Geometry: final body of the model. Coordinates: model frame, mm. A direction names the side the tool comes from. Round coordinates to 2 decimals unless told otherwise and drop trailing zeros. Loops run counter-clockwise (first coordinate to the right, second up) from the corner with the lowest first, then second, coordinate; pieces in that order, holes last. Notation, with made-up numbers: (24, 79.5) - (50, 79.5) arc R20 cw to (50, 87.5) - close; hole circle Ø7 at (3, 66). An arc over 180 degrees is marked (long way). Return JSON: item names as keys, results as strings. Group by question number.
1. Draft query along X for faces 1 (the face through (-11.99, 0.53, 11.75)), 2 (the face through (-2, 14, 13)), 3 (the face through (138.75, 4, 12)). Return one class per face: +X half, -X half, draft (parallel to the pull), parting line (faces both ways), or undercut.
2. Section B-B on x = -62.5. Return loops of the section in (y, z).
3. Section A-A on z = 10.1. Return loops of the section in (x, y), and give its area (3 significant figures).
4. First-contact query: pin 1 Ø2 at (x, z) = (31.5, 9.5) entering from -Y; pin 2 Ø2 at (x, y) = (-41.25, -58) entering from -Z; pin 3 Ø1.3 at (x, z) = (52, 8.5) entering from +Y. Flat tips, straight axial feed; report the tip coordinate or a pass-through.
5. Material intervals for probe 1 along X at (y, z) = (58, 11.75); probe 2 along Y at (x, z) = (-41.25, 11.7); probe 3 along Y at (x, z) = (-21, 7.35), sorted ascending.
6. Section C-C on y = 23. Return loops of the section in (x, z), and give its area (3 significant figures).
7. Set-up query: faces 4 (the face through (-2, 51, 11.5)), 5 (the face through (-138.75, 4, 12)), 6 (the face through (-2, 18, 11.5)), 7 (the face through (-2, -50, 11.5)). Return all of +Z, -Z, +X, -X, +Y, -Y with unobstructed straight access to the full face (end or side cutting, diameter ignored); none if empty.
from build123d import *

# Parameters (mm, degrees)
SKETCH017_W     = 277.5
SKETCH017_H     = 121
PAD007_DEPTH    = 1.5
SKETCH018_R     = 0.9
POCKET006_DEPTH = 1.501
SKETCH025_W     = 277.5
SKETCH025_H     = 2
PAD009_DEPTH    = 4.5
SKETCH026_R     = 12
POCKET007_DEPTH = 6.001
CHAMFER_SIZE    = 1


with BuildPart() as part:
    # Sketch017 → Pad007 (new body)
    with BuildSketch(Plane.XY.offset(13)):
        Rectangle(SKETCH017_W, SKETCH017_H)
    extrude(amount=-PAD007_DEPTH)

    # Sketch018 (on Face6 of Pad007) → Pocket006 (cut, through all)
    with BuildSketch(Plane(origin=(0, 0, 11.5), x_dir=(1, 0, 0), z_dir=(0, 0, -1))):
        with Locations((-135.25, 58)):
            Circle(SKETCH018_R)
        with Locations((-41.25, 58)):
            Circle(SKETCH018_R)
        with Locations((-31.25, 58)):
            Circle(SKETCH018_R)
        with Locations((43.75, 58)):
            Circle(SKETCH018_R)
        with Locations((135.25, 58)):
            Circle(SKETCH018_R)
        with Locations((135.25, -58)):
            Circle(SKETCH018_R)
        with Locations((43.75, -58)):
            Circle(SKETCH018_R)
        with Locations((-31.25, -58)):
            Circle(SKETCH018_R)
        with Locations((-41.25, -58)):
            Circle(SKETCH018_R)
        with Locations((-135.25, -58)):
            Circle(SKETCH018_R)
    extrude(amount=-POCKET006_DEPTH, mode=Mode.SUBTRACT)

    # Sketch025 (on Face5 of Pocket006) → Pad009 (join)
    with BuildSketch(Plane(origin=(0, 0, 11.5), x_dir=(1, 0, 0), z_dir=(0, 0, -1))):
        with Locations((0, 39.5)):
            Rectangle(SKETCH025_W, SKETCH025_H)
        with Locations((0, -39.5)):
            Rectangle(SKETCH025_W, SKETCH025_H)
    extrude(amount=PAD009_DEPTH)

    # Sketch026 (on Face2 of Pad009) → Pocket007 (cut, through all)
    with BuildSketch(Plane.XY.offset(13)):
        Circle(SKETCH026_R)
    extrude(amount=-POCKET007_DEPTH, mode=Mode.SUBTRACT)

    # Chamfer
    chamfer_edges = [part.edges().sort_by_distance(p)[0] for p in [
        (134.35, -58, 13),
        (42.85, -58, 13),
        (-32.15, -58, 13),
        (-42.15, -58, 13),
        (-136.15, -58, 13),
        (-136.15, 58, 13),
        (-42.15, 58, 13),
        (-32.15, 58, 13),
        (42.85, 58, 13),
        (134.35, 58, 13),
        (-12, 0, 13),
    ]]
    chamfer(chamfer_edges, length=CHAMFER_SIZE)


solid = part.part
Taken from the geometry:
{
 "1": {"face 1": "undercut", "face 2": "draft", "face 3": "+X half"},
 "2": {"outline": "(-60.5, 11.5) - (-40.5, 11.5) - (-40.5, 7) - (-38.5, 7) - (-38.5, 11.5) - (38.5, 11.5) - (38.5, 7) - (40.5, 7) - (40.5, 11.5) - (60.5, 11.5) - (60.5, 13) - (-60.5, 13) - close"},
 "3": {"outline": "(-138.75, -40.5) - (138.75, -40.5) - (138.75, -38.5) - (-138.75, -38.5) - close; (-138.75, 38.5) - (138.75, 38.5) - (138.75, 40.5) - (-138.75, 40.5) - close", "area": "1,110 mm2"},
 "4": {"pin 1": "y = -40.5", "pin 2": "z = 11.5", "pin 3": "y = 40.5"},
 "5": {"probe 1": "-138.75 to -136.15, -134.35 to -42.15, -40.35 to -32.15, -30.35 to 42.85, 44.65 to 134.35, 136.15 to 138.75", "probe 2": "-60.5 to -58.9, -57.1 to 57.1, 58.9 to 60.5", "probe 3": "-40.5 to -38.5, 38.5 to 40.5"},
 "6": {"outline": "(-138.75, 11.5) - (138.75, 11.5) - (138.75, 13) - (-138.75, 13) - close", "area": "416 mm2"},
 "7": {"face 4": "-Z, +X, -X, +Y", "face 5": "+Z, -Z, -X, +Y, -Y", "face 6": "-Z, +X, -X", "face 7": "-Z, +X, -X, -Y"}
}
